The model under review builds one solid part; all positions refer to its coordinate system, in mm. A direction names the side the tool comes from. Coordinates: 2 decimals unless noted, no trailing zeros. Write each loop counter-clockwise with the first axis right and the second up, starting at its lowest first coordinate (ties: lowest second). Pieces come first, ordered by that corner, then holes.
```python
from build123d import *

# Parameters (mm, degrees)
F0_W      = 50.8
F0_H      = 55.88
F1_DEPTH  = 5.08
F2_W      = 50.8
F2_H      = 5.08
F3_DEPTH  = 20.32
F4_W      = 50.8
F4_H      = 5.08
F5_DEPTH  = 53.975
F6_W      = 50.8
F6_H      = 5.08
F7_DEPTH  = 50.8
F8_W      = 12.7
F8_H      = 20.32
F9_DEPTH  = 31.75
F10_W     = 25.4
F10_H     = 7.62
F11_DEPTH = 50.8


with BuildPart() as f1:
    # F0 (on Top) → F1 (new body)
    with BuildSketch(Plane.XY):
        with Locations((25.4, 27.94)):
            Rectangle(F0_W, F0_H)
    extrude(amount=F1_DEPTH)

    # F2 (on face) → F3 (join)
    with BuildSketch(Plane(origin=(0, 0, 0), x_dir=(1, 0, 0), z_dir=(0, 0, -1))):
        with Locations((25.4, -53.34)):
            Rectangle(F2_W, F2_H)
    extrude(amount=F3_DEPTH)

    # F4 (on face) → F5 (join)
    with BuildSketch(Plane.XZ.offset(-50.8)):
        with Locations((25.4, -17.78)):
            Rectangle(F4_W, F4_H)
    extrude(amount=F5_DEPTH)

    # F6 (on face) → F7 (join)
    with BuildSketch(Plane(origin=(0, 0, -20.32), x_dir=(1, 0, 0), z_dir=(0, 0, -1))):
        with Locations((25.4, 0.635)):
            Rectangle(F6_W, F6_H)
    extrude(amount=F7_DEPTH)

    # F8 (on face) → F9 (join)
    with BuildSketch(Plane(origin=(0, 1.905, 0), x_dir=(-1, 0, 0), z_dir=(0, 1, 0))):
        with Locations((-44.45, -60.96)):
            Rectangle(F8_W, F8_H)
        with Locations((-6.35, -60.96)):
            Rectangle(F8_W, F8_H)
    extrude(amount=F9_DEPTH)

    # F10 (on face) → F11 (cut)
    with BuildSketch(Plane.YZ.offset(50.8)):
        with Locations((14.605, -54.61)):
            Rectangle(F10_W, F10_H)
    extrude(amount=-F11_DEPTH, mode=Mode.SUBTRACT)


solid = f1.part
```
Item 1: Mouldability with a two-part tool opening along Y and no side actions: class faces 6 (the face through (25, 24, -15.24)), 7 (the face through (45, 33.655, -61)), 8 (the face through (45, 14, -58.42)) as pulls with the +Y half, pulls with the -Y half, needs draft (parallel to the pull), parting line crosses it, or undercut.
Solved:
face 6: needs draft
face 7: pulls with the +Y half
face 8: undercut
Item 2: Machinability: for faces 1 (the face through (6, 14, -58.42)), 2 (the face through (6, 30, -50.8)), 3 (the face through (25, 26, 0)), 4 (the face through (6, 33.655, -61)), 5 (the face through (25, 0, 3)), which of the approach directions +Z, -Z, +X, -X, +Y, -Y give a long, thin tool a straight path to every point of the face, cutting with its end or side? Answer none if there is none.
Solved:
face 1: +X, -X
face 2: +X, -X, +Y
face 3: +X, -X, -Y
face 4: -Z, +X, -X, +Y
face 5: +Z, +X, -X, -Y
Item 3: To check wall thickness, follow line 1 along Z through (x, y) = (9, 24.5); line 2 along Z through (x, y) = (31, 32.5); line 3 along X through (y, z) = (31, -52.5). State the ranges of each line that lie inside material, in increasing order.
Solved:
line 1: z = -71.12 to -58.42, -20.32 to -15.24, 0 to 5.08
line 2: z = -20.32 to -15.24, 0 to 5.08
line 3: x = 0 to 12.7, 38.1 to 50.8
Item 4: Take a section at A-A, the plane y = 35. Write out the cut boundary in (x, z), plus the area to 3 significant figures.
Solved:
outline: (0, -20.32) - (50.8, -20.32) - (50.8, -15.24) - (0, -15.24) - close; (0, 0) - (50.8, 0) - (50.8, 5.08) - (0, 5.08) - close
area: 516 mm2
Item 5: Take a section at D-D, the plane y = 6. Write out the cut boundary in (x, z).
Solved:
outline: (0, -71.12) - (12.7, -71.12) - (12.7, -58.42) - (0, -58.42) - close; (0, -20.32) - (50.8, -20.32) - (50.8, -15.24) - (0, -15.24) - close; (0, 0) - (50.8, 0) - (50.8, 5.08) - (0, 5.08) - close; (38.1, -71.12) - (50.8, -71.12) - (50.8, -58.42) - (38.1, -58.42) - close
Item 6: For pin 1 (2 mm diameter, centred on x = 28, z = -6, fed in from -Y); pin 2 (4 mm diameter, centred on x = 44, z = -63, fed in from +Y) (3 decimals); pin 3 (5 mm diameter, centred on x = 35, z = -53, fed in from +Y) (3 decimals), all flat-tipped, find the tip position at first contact; note any pin that passes through.
Solved:
pin 1: stops at y = 50.8
pin 2: stops at y = 33.655
pin 3: stops at y = 1.905
Item 7: Take a section at B-B, the plane z = -57. Write out the cut boundary in (x, y) (3 decimals), plus the area to 3 significant figures.
Solved:
outline: (0, -3.175) - (50.8, -3.175) - (50.8, 1.905) - (0, 1.905) - close; (0, 27.305) - (12.7, 27.305) - (12.7, 33.655) - (0, 33.655) - close; (38.1, 27.305) - (50.8, 27.305) - (50.8, 33.655) - (38.1, 33.655) - close
area: 419 mm2
Item 8: Take a section at C-C, the plane x = 24. Write out the cut boundary in (y, z) (3 decimals), plus the area to 3 significant figures.
Solved:
outline: (-3.175, -71.12) - (1.905, -71.12) - (1.905, -20.32) - (55.88, -20.32) - (55.88, 5.08) - (0, 5.08) - (0, 0) - (50.8, 0) - (50.8, -15.24) - (-3.175, -15.24) - close
area: 919 mm2
